Geometry: final body of the model. Coordinates: model frame, mm. A direction names the side the tool comes from. Coordinates: 2 decimals unless noted, no trailing zeros. Order: outer loops, then holes, each group sorted by start corner. A loop starts at its lowest first (then second) coordinate and runs counter-clockwise, first axis right, second up. Notation, with made-up numbers: (85.25, -27) -> (138.25, -27) arc R33 ccw to (138.25, 12) -> close; hole circle Ø10 at (78.25, 78). An arc over 180 degrees is marked (long way). Answer in a Markdown table with one row per item. Add a question column.
1) Section query B-B on x = 0. Return the cut outline in (y, z).
2) Ray query, line 1 (X direction, y = -4.5, z = 12.5); line 2 (Z direction, x = 5, y = 0); line 3 (Y direction, x = 0, z = 2). Return the intervals inside material, ascending. Write a range as from..to.
3) Section query D-D on x = 5. Return the cut outline in (y, z).
4) Contact query for flat-ended pins moving along their axis: P1, Ø1.5, axis at x = -2.5, z = 10.5, coming from the -Y side; P2, Ø2, axis at y = 0.5, z = 15.5, coming from the -X side; P3, Ø5.5, axis at x = 6, z = 10.5, coming from the +Y side; P4, Ø6, axis at y = -12, z = 16, coming from the +X side. Output: stop coordinate, or through.
5) Set-up query: faces 1 (the face through (-7.5, 0, 9)), 2 (the face through (-5, 7.5, 9)), 3 (the face through (7.5, 0, 9)), 4 (the face through (-5, -7.5, 9)), 5 (the face through (-2.5, 0, 9)). Return all of +Z, -Z, +X, -X, +Y, -Y with unobstructed straight access to the full face (end or side cutting, diameter ignored); none if empty.
6) Section query C-C on y = -1.5. Return the cut outline in (x, z).
7) Section query A-A on z = 11. Return the cut outline in (x, y), then the cut area to 3 significant figures.
8) Pull-direction query (Y, two-part tool) for faces 6 (the face through (5.04, -0.54, 10.06)), 7 (the face through (2.5, 0, 9)), 8 (the face through (5, 7.5, 9)), 9 (the face through (5, -7.5, 9)); classes: +Y half, -Y half, draft (parallel to the pull), parting line (faces both ways), or undercut.
```python
from build123d import *

# Parameters (mm, degrees)
CROQUIS1_R              = 20
SALIENTE_EXTRUIR1_DEPTH = 5
CROQUIS2_R              = 2.5
CORTAR_EXTRUIR1_DEPTH   = 5
CROQUIS3_W              = 5
CROQUIS3_H              = 15
SALIENTE_EXTRUIR3_DEPTH = 15
CROQUIS4_R              = 2.5
CORTAR_EXTRUIR2_DEPTH   = 5


with BuildPart() as part:
    # Croquis1 → Saliente-Extruir1 (new body)
    with BuildSketch(Plane.XY):
        Circle(CROQUIS1_R)
    extrude(amount=SALIENTE_EXTRUIR1_DEPTH)

    # Croquis2 → Cortar-Extruir1 (cut)
    with BuildSketch(Plane.XY.offset(5)):
        Circle(CROQUIS2_R)
    extrude(amount=-CORTAR_EXTRUIR1_DEPTH, mode=Mode.SUBTRACT)

    # Croquis3 → Saliente-Extruir3 (add)
    with BuildSketch(Plane.XY.offset(5)):
        with Locations((5, 0)):
            Rectangle(CROQUIS3_W, CROQUIS3_H)
    extrude(amount=SALIENTE_EXTRUIR3_DEPTH)

    # Croquis4 → Cortar-Extruir2 (cut)
    with BuildSketch(Plane(origin=(7.5, 0, 0), x_dir=(0, 0, -1), z_dir=(1, 0, 0))):
        with BuildLine():
            ThreePointArc((-12.5, -7.5), (-17.803300859, -5.303300859), (-20, 0))
            Line((-20, 0), (-20, -7.5))
            Line((-20, -7.5), (-12.5, -7.5))
        make_face()
        with BuildLine():
            ThreePointArc((-20, 0), (-17.803300859, 5.303300859), (-12.5, 7.5))
            Line((-12.5, 7.5), (-20, 7.5))
            Line((-20, 7.5), (-20, 0))
        make_face()
        with Locations(Location((-12.5, 0, 0), (0, 0, 90))):
            Circle(CROQUIS4_R)
    extrude(amount=-CORTAR_EXTRUIR2_DEPTH, mode=Mode.SUBTRACT)

    # Simetría1: part across plane


with BuildPart() as part_1:
    add(part.part)
    add(part.part.mirror(Plane(origin=(0, 0, 0), x_dir=(0, 0, 1), z_dir=(1, 0, 0))))


solid = part_1.part
```
Result:
| question | item | result |
|---|---|---|
| 1 | outline | (-20, 0) -> (-2.5, 0) -> (-2.5, 5) -> (-20, 5) -> close; (2.5, 0) -> (20, 0) -> (20, 5) -> (2.5, 5) -> close |
| 2 | line 1 | -7.5..-2.5, 2.5..7.5 |
| 2 | line 2 | 0..10, 15..20 |
| 2 | line 3 | -20..-2.5, 2.5..20 |
| 3 | outline | (-19.36, 0) -> (19.36, 0) -> (19.36, 5) -> (7.5, 5) -> (7.5, 12.5) arc R7.5 ccw to (-7.5, 12.5) -> (-7.5, 5) -> (-19.36, 5) -> close; hole circle Ø5 at (0, 12.5) |
| 4 | P1 | y = -7.5 |
| 4 | P2 | x = -7.5 |
| 4 | P3 | y = 7.5 |
| 4 | P4 | through |
| 5 | face 1 | +Z, -X, +Y, -Y |
| 5 | face 2 | +Z, +X, -X, +Y |
| 5 | face 3 | +Z, +X, +Y, -Y |
| 5 | face 4 | +Z, +X, -X, -Y |
| 5 | face 5 | +Z, +Y, -Y |
| 6 | outline | (-19.94, 0) -> (-2, 0) -> (-2, 5) -> (-2.5, 5) -> (-2.5, 10.5) -> (-7.5, 10.5) -> (-7.5, 5) -> (-19.94, 5) -> close; (-7.5, 14.5) -> (-2.5, 14.5) -> (-2.5, 19.85) -> (-7.5, 19.85) -> close; (2, 0) -> (19.94, 0) -> (19.94, 5) -> (7.5, 5) -> (7.5, 10.5) -> (2.5, 10.5) -> (2.5, 5) -> (2, 5) -> close; (2.5, 14.5) -> (7.5, 14.5) -> (7.5, 19.85) -> (2.5, 19.85) -> close |
| 7 | outline | (-7.5, -7.5) -> (-2.5, -7.5) -> (-2.5, -2) -> (-7.5, -2) -> close; (-7.5, 2) -> (-2.5, 2) -> (-2.5, 7.5) -> (-7.5, 7.5) -> close; (2.5, -7.5) -> (7.5, -7.5) -> (7.5, -2) -> (2.5, -2) -> close; (2.5, 2) -> (7.5, 2) -> (7.5, 7.5) -> (2.5, 7.5) -> close |
| 7 | area | 110 mm2 |
| 8 | face 6 | undercut |
| 8 | face 7 | draft |
| 8 | face 8 | +Y half |
| 8 | face 9 | -Y half |
